```python
from build123d import *

# Parameters (mm, degrees)
SKETCH1_R           = 11
BOSS_EXTRUDE1_DEPTH = 3.15
CHAMFER1_SIZE       = 1.25


with BuildPart() as part:
    # Sketch1 → Boss-Extrude1 (new body)
    with BuildSketch(Plane.XY):
        Circle(SKETCH1_R)
        Polygon((8.371578903, 0), (4.185789452, 7.25), (-4.185789452, 7.25), (-8.371578903, 0), (-4.185789452, -7.25), (4.185789452, -7.25), align=None, mode=Mode.SUBTRACT)
    extrude(amount=BOSS_EXTRUDE1_DEPTH)

    # Chamfer1
    chamfer1_edges = [part.edges().sort_by_distance(p)[0] for p in [
        (-11, 0, 0),
    ]]
    chamfer(chamfer1_edges, length=CHAMFER1_SIZE)


solid = part.part
```
CAD build for the part. Positions are in the model's coordinates, mm. A direction names the side the tool comes from. Round coordinates to 2 decimals unless told otherwise and drop trailing zeros. Write each loop counter-clockwise with the first axis right and the second up, starting at its lowest first coordinate (ties: lowest second). Pieces come first, ordered by that corner, then holes. Notation, with made-up numbers: M 46,-5 L 69,-5 A12 ccw 69,3 Z; hole C 32.5,-21 d9. An arc over 180 degrees is marked long. One line per question, with ' | ' between items.
1. Pin check, flat tips, straight feed: pin 1 Ø1.5 at (x, z) = (-5, 1) entering from +Y; pin 2 Ø1.5 at (x, z) = (6.5, 0.5) entering from -Y; pin 3 Ø4 at (x, y) = (-4.5, -2) entering from +Z. Stop position of each tip, or through.
Working result:
pin 1: y = 10.13 | pin 2: y = -9.02 | pin 3: through
2. Cut at C-C on z = 0.3. Write the cut outline in (x, y).
Working result:
outline: C 0,0 d20.1; hole M -8.37,0 L -4.19,-7.25 L 4.19,-7.25 L 8.37,0 L 4.19,7.25 L -4.19,7.25 Z
3. Which spindle directions (+Z, -Z, +X, -X, +Y, -Y) get a long thin tool onto all of the face, cutting with end or side? Do faces 1 (the flat face through (-6.31, -3.57, 1.55)), 2 (the flat face through (6.5, 3.7, 0)). Say none if no direction does.
Working result:
face 1: +Z, -Z | face 2: -Z, +X, -X, +Y, -Y
4. Mould opens along X. For faces 3 (the flat face through (-6.249, 3.676, 1.553)), 4 (the cylindrical face through (-2.38, -10.74, 2.19)), 5 (the flat face through (7, 3, 3.15)) say: pulls with the +X half, pulls with the -X half, needs draft (parallel to the pull), parting line crosses it, or undercut.
Working result:
face 3: undercut | face 4: parting line crosses it | face 5: needs draft
5. Probe L1, parallel to Y at x = -1.25, z = 0.25; L2, parallel to X at y = -3.25, z = 2.4; L3, parallel to Y at x = -1.5, z = 2.85. List the from-to ranges inside material, lowest first. Write a range as from..to.
Working result:
L1: -9.92..-7.25, 7.25..9.92 | L2: -10.51..-6.5, 6.5..10.51 | L3: -10.9..-7.25, 7.25..10.9
6. Cut at B-B on x = 0. Write the cut outline in (y, z).
Working result:
outline: M -11,1.25 L -9.75,0 L -7.25,0 L -7.25,3.15 L -11,3.15 Z; M 7.25,0 L 9.75,0 L 11,1.25 L 11,3.15 L 7.25,3.15 Z
7. Cut at A-A on z = 2.5. Write the cut outline in (x, y).
Working result:
outline: C 0,0 d22; hole M -8.37,0 L -4.19,-7.25 L 4.19,-7.25 L 8.37,0 L 4.19,7.25 L -4.19,7.25 Z
